CAD build for the part. Positions are in the model's coordinates, mm. A direction names the side the tool comes from. Round coordinates to 2 decimals unless told otherwise and drop trailing zeros. Loops run counter-clockwise (first coordinate to the right, second up) from the corner with the lowest first, then second, coordinate; pieces in that order, holes last. Notation, with made-up numbers: M -10,31.25 L 38,31.25 A18 cw 38,41.25 Z; hole C -29,69.25 d9. An arc over 180 degrees is marked long. Use a Markdown table: item, result. Add a question column.
(1) Wall check: L1, parallel to X at y = -22.25, z = -31.5; L2, parallel to Z at x = -7, y = -8.5; L3, parallel to Y at x = 17, z = -28. Give the ranges that are in metal, low to high.
(2) Band-saw the part on C-C, the plane x = -10.5. Write the cut outline in (y, z), and give its area (3 significant figures).
(3) Flat gauge pin, fed straight in: P1, Ø6, axis at x = -26, z = 4.5, coming from the -Y side. Where does the tip first touch, or does it go through?
(4) Band-saw the part on A-A, the plane z = 17.5. Write the cut outline in (x, y).
(5) Two-plate mould, pull along Z, no slides. Class faces 3 (the face through (0, 0, -5)), 4 (the face through (1, -13, 24.577)), 5 (the face through (50.62, -14, -5)): released by +Z, released by -Z, zero draft, split by the parting line, or undercut.
(6) Which spindle directions (+Z, -Z, +X, -X, +Y, -Y) get a long thin tool onto all of the face, cutting with end or side? Do faces 1 (the face through (0, -14, -31.997)), 2 (the face through (-4, -25.4, -33)). Say none if no direction does.
(7) Band-saw the part on B-B, the plane y = -20.5. Write the cut outline in (x, z), and give its area (3 significant figures).
from build123d import *

# Parameters (mm, degrees)
F1_DEPTH = 25.4
F2_T     = -2.54


with BuildPart() as f1:
    # F0 (on Front) → F1 (new body)
    with BuildSketch(Plane.XZ):
        Polygon((-32.8051820397, 24.5768204331), (-52.0768724382, 24.5768204331), (-52.0768724382, -34.5374681056), (-21.7618532479, -34.5374681056), align=None)
        Polygon((53.1595535576, 24.5768204331), (-32.8051820397, 24.5768204331), (-21.7618532479, -34.5374681056), (53.1595535576, -34.5374681056), align=None)
    extrude(amount=F1_DEPTH)

    # F2
    f2_openings = [f1.faces().sort_by_distance(p)[0] for p in [
        (0.541341, -25.4, -4.980324),
    ]]
    offset(amount=F2_T, openings=f2_openings)


solid = f1.part
Return value:
| question | item | result |
|---|---|---|
| 1 | L1 | -52.08 to -49.54, 50.62 to 53.16 |
| 1 | L2 | -34.54 to -32, 22.04 to 24.58 |
| 1 | L3 | -2.54 to 0 |
| 2 | outline | M -25.4,-34.54 L 0,-34.54 L 0,24.58 L -25.4,24.58 L -25.4,22.04 L -2.54,22.04 L -2.54,-32 L -25.4,-32 Z |
| 2 | area | 266 mm^2 |
| 3 | P1 | y = -2.54 |
| 4 | outline | M -52.08,-25.4 L -49.54,-25.4 L -49.54,-2.54 L 50.62,-2.54 L 50.62,-25.4 L 53.16,-25.4 L 53.16,0 L -52.08,0 Z |
| 5 | face 3 | zero draft |
| 5 | face 4 | released by +Z |
| 5 | face 5 | undercut |
| 6 | face 1 | -Y |
| 6 | face 2 | +Z, -Z, +X, -X, -Y |
| 7 | outline | M -52.08,-34.54 L 53.16,-34.54 L 53.16,24.58 L -52.08,24.58 Z; hole M -49.54,-32 L 50.62,-32 L 50.62,22.04 L -49.54,22.04 Z |
| 7 | area | 809 mm^2 |
